```python
from build123d import *

# Parameters (mm, degrees)
BASE_FLANGE2_DEPTH = 40
SKETCH11_R         = 3
CUT_EXTRUDE2_DEPTH = 10
SKETCH12_R         = 12
SKETCH12_R_2       = 3
CUT_EXTRUDE3_DEPTH = 10


# Sheet-metal steps are written as plain solids
with BuildPart() as part:
    # Sketch1 → Base-Flange2 (new body)
    with BuildSketch(Plane.XY):
        with BuildLine():
            Line((0, 18), (0, 2))
            ThreePointArc((0, 2), (0.585786438, 0.585786438), (2, 0))
            Line((2, 0), (18, 0))
            Line((18, 0), (18, -2))
            Line((18, -2), (2, -2))
            ThreePointArc((2, -2), (-0.828427125, -0.828427125), (-2, 2))
            Line((-2, 2), (-2, 18))
            Line((-2, 18), (0, 18))
        make_face()
    extrude(amount=BASE_FLANGE2_DEPTH)

    # Sketch11 → Cut-Extrude2 (cut)
    with BuildSketch(Plane(origin=(0, 0, 0), x_dir=(0, 0, -1), z_dir=(1, 0, 0))):
        with Locations((-32, 12)):
            Circle(SKETCH11_R)
        with Locations((-8, 12)):
            Circle(SKETCH11_R)
    extrude(amount=-CUT_EXTRUDE2_DEPTH, mode=Mode.SUBTRACT)

    # Sketch12 → Cut-Extrude3 (cut)
    with BuildSketch(Plane(origin=(0, 0, 0), x_dir=(1, 0, 0), z_dir=(0, 1, 0))):
        with Locations((23, -20)):
            Circle(SKETCH12_R)
        with Locations(Location((10, -8, 0), (0, 0, 270))):
            Circle(SKETCH12_R_2)
        with Locations(Location((10, -32, 0), (0, 0, 270))):
            Circle(SKETCH12_R_2)
    extrude(amount=-CUT_EXTRUDE3_DEPTH, mode=Mode.SUBTRACT)


solid = part.part
```
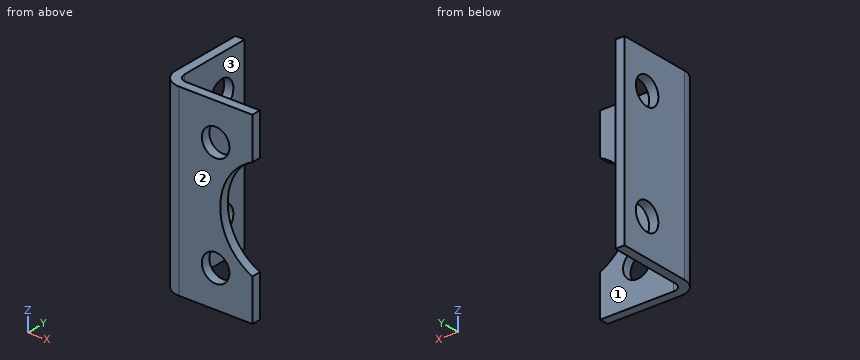
The listing builds one solid part. Answer for the finished solid, in the listing's coordinates (mm). Face numbers are marked on the shaded views. Round coordinates to 2 decimals unless told otherwise and drop trailing zeros. Write each loop counter-clockwise with the first axis right and the second up, starting at its lowest first coordinate (ties: lowest second). Pieces come first, ordered by that corner, then holes. Notation, with made-up numbers: (-16, 23) -> (14, 23) arc R17 cw to (14, 51) -> close; hole circle Ø11 at (68, 27). An arc over 180 degrees is marked (long way). Answer as a JSON object with one key per item and string values. Group by question number.
Q1. Straight lines are drawn through the part: line 1 along X through (y, z) = (5.5, 38.5); line 2 along X through (y, z) = (-0.5, 8). For each, find the intervals that lie inside material, in ascending order.
Q2. Each of these flat-tipped pins is pushed along its axis until it touches: pin 1 Ø4 at (x, z) = (13.5, 26.5) entering from +Y; pin 2 Ø3.5 at (y, z) = (12, 32) entering from +X; pin 3 Ø7 at (y, z) = (12, 8) entering from +X. Where does it stop, or does it pass through?
Q3. Section B-B (x = 10) is taken. Write down the section's boundary in (y, z), plus the area to 3 significant figures.
Q4. Section D-D (x = 15.75) is taken. Write down the section's boundary in (y, z), plus the area to 3 significant figures.
Q5. Section A-A (z = 8) is taken. Write down the section's boundary in (x, y).
Q6. Determine the mould class of the marked faces 1, 2 and 3 for opening direction Y: pulls with the +Y half, pulls with the -Y half, needs draft (parallel to the pull), parting line crosses it, or undercut.
Check values:
{
 "1": {"line 1": "-2 to 0", "line 2": "-1.12 to 7, 13 to 18"},
 "2": {"pin 1": "y = 0", "pin 2": "through", "pin 3": "x = 0"},
 "3": {"outline": "(-2, 0) -> (0, 0) -> (0, 5) -> (-2, 5) -> close; (-2, 11) -> (0, 11) -> (0, 29) -> (-2, 29) -> close; (-2, 35) -> (0, 35) -> (0, 40) -> (-2, 40) -> close", "area": "56.0 mm^2"},
 "4": {"outline": "(-2, 0) -> (0, 0) -> (0, 10.44) -> (-2, 10.44) -> close; (-2, 29.56) -> (0, 29.56) -> (0, 40) -> (-2, 40) -> close", "area": "41.8 mm^2"},
 "5": {"outline": "(-2, 2) arc R4 ccw to (2, -2) -> (7, -2) -> (7, 0) -> (2, 0) arc R2 cw to (0, 2) -> (0, 9) -> (-2, 9) -> close; (-2, 15) -> (0, 15) -> (0, 18) -> (-2, 18) -> close; (13, -2) -> (18, -2) -> (18, 0) -> (13, 0) -> close"},
 "6": {"face 1": "pulls with the +Y half", "face 2": "pulls with the -Y half", "face 3": "needs draft"}
}
